Part print with two shaded views. Sizes in mm from the minimum x, y, z corner. A direction names the side the tool comes from. Give positions to 0.01 mm unless a question says otherwise; leave off trailing zeros. Loops run counter-clockwise (first coordinate to the right, second up) from the corner with the lowest first, then second, coordinate; pieces in that order, holes last. Notation, with made-up numbers: M -5.5,82.5 L 42.5,82.5 A26 cw 42.5,104.5 Z; hole C -27.5,21 d4. An arc over 180 degrees is marked long. Answer as a JSON object with one key per item and string values. Group by question number.
1. 3-axis set-ups, long thin cutter, end or side, ignore diameter. For the marked faces 4 and 5: which of +Z, -Z, +X, -X, +Y, -Y reach the whole face in a straight line?
2. Drop flat-ended pins along their axis: pin 1 Ø4 at (y, z) = (53, 18.5) entering from -X; pin 2 Ø3.5 at (x, z) = (15.875, 44.45) entering from +Y; pin 3 Ø6 at (x, z) = (12, 7) entering from -Y. Give the stop position or say it passes through.
3. Slice it at A-A (x = 31.75). List the corners of the cut face in (y, z), then the cut area to 3 significant figures.
4. Slice it at B-B (y = 12.7). Give the number of separate pieces and of enclosed holes in the cut face, then the cut area to 3 significant figures.
5. Mould opens along Y. For the marked faces 1, 2 and 3 say: released by +Y, released by -Y, zero draft, split by the parting line, or undercut.
6. Drill centre lines: line 1 along X through (y, z) = (61.25, 44.45) (1 decimal); line 2 along Y through (x, z) = (59, 25.4); line 3 along X through (y, z) = (59, 44). Where is each one in solid material? Low to high. Write a range as [from, to].
7. Slice it at D-D (z = 25.4). List the corners of the cut face in (x, y).
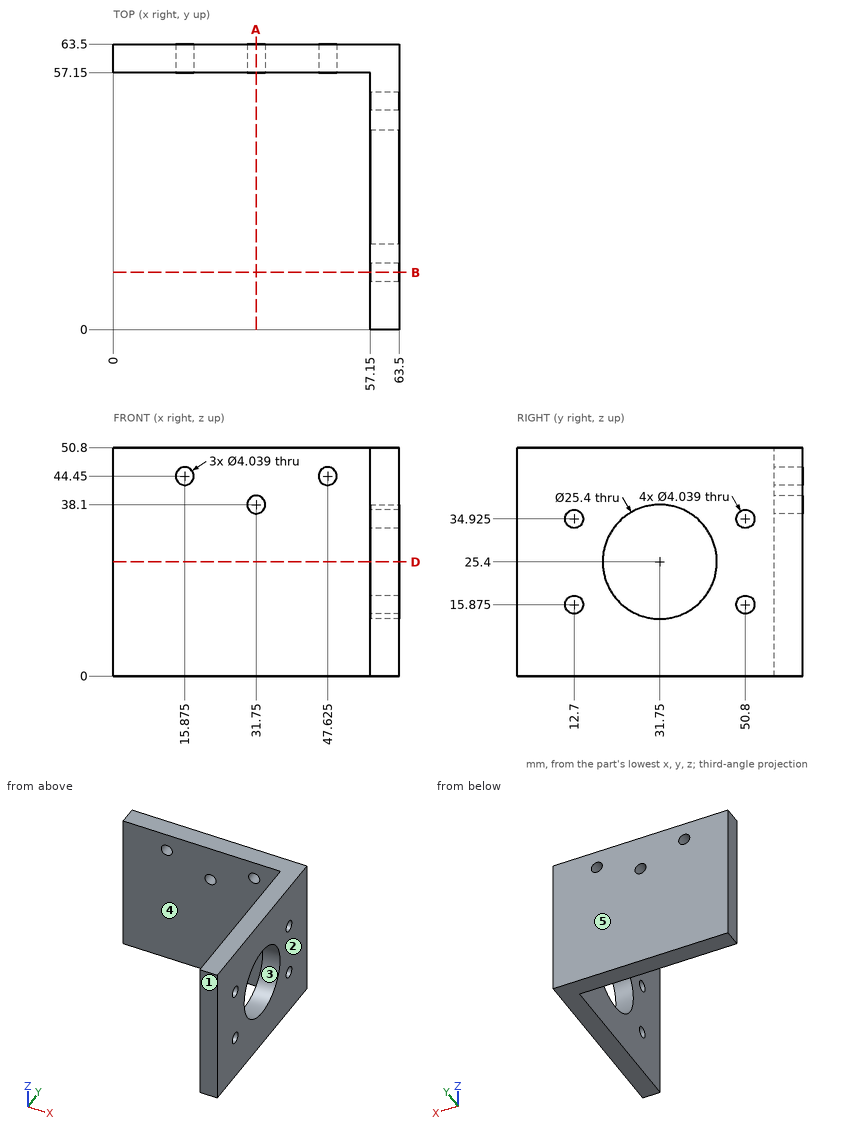
Established:
{
 "1": {"face 4": "+Z, -Z, -X, -Y", "face 5": "+Z, -Z, +X, -X, +Y"},
 "2": {"pin 1": "stops at x = 57.15", "pin 2": "passes through", "pin 3": "stops at y = 57.15"},
 "3": {"outline": "M 57.15,0 L 63.5,0 L 63.5,36.08 L 57.15,36.08 Z; M 57.15,40.12 L 63.5,40.12 L 63.5,50.8 L 57.15,50.8 Z", "area": "297 mm^2"},
 "4": {"separate pieces": "3", "enclosed holes": "0", "area": "271 mm^2"},
 "5": {"face 1": "released by -Y", "face 2": "zero draft", "face 3": "undercut"},
 "6": {"line 1": "x = [0, 13.9], [17.9, 45.6], [49.6, 63.5]", "line 2": "y = [0, 19.05], [44.45, 63.5]", "line 3": "x = [0, 13.91], [17.84, 45.66], [49.59, 63.5]"},
 "7": {"outline": "M 0,57.15 L 57.15,57.15 L 57.15,44.45 L 63.5,44.45 L 63.5,63.5 L 0,63.5 Z; M 57.15,0 L 63.5,0 L 63.5,19.05 L 57.15,19.05 Z"}
}
